Verification items for the finished model (mm, model axes). A direction names the side the tool comes from. Round coordinates to 2 decimals unless told otherwise and drop trailing zeros. Loops run counter-clockwise (first coordinate to the right, second up) from the corner with the lowest first, then second, coordinate; pieces in that order, holes last. Notation, with made-up numbers: (32, -36.5) -> (87, -36.5) arc R20 ccw to (87, -24.5) -> close; hole circle Ø11 at (-14, -1). An arc over 180 degrees is marked (long way). Write item = value, one per line. Start each with the question number.
```python
from build123d import *

# Parameters (mm, degrees)
SKETCH2_R           = 15
SKETCH2_R_2         = 11
BOSS_EXTRUDE1_DEPTH = 9
BOSS_EXTRUDE2_DEPTH = 9
SKETCH4_W           = 12.7
SKETCH4_H           = 16
BOSS_EXTRUDE3_DEPTH = 3.8
SKETCH5_R           = 1.275
CUT_EXTRUDE1_DEPTH  = 7
SKETCH6_R           = 11
SKETCH6_R_2         = 8
BOSS_EXTRUDE4_DEPTH = 1.5
BOSS_EXTRUDE5_DEPTH = 9
SKETCH8_W           = 12
SKETCH8_H           = 2
SKETCH8_W_2         = 2
SKETCH8_H_2         = 12
CUT_EXTRUDE2_DEPTH  = 13.8
CUT_EXTRUDE3_REACH  = 34
SKETCH9_R           = 0.95
CUT_EXTRUDE4_REACH  = 48.456
SKETCH10_R          = 0.95
FILLET1_R           = 4
FILLET3_R           = 2
SKETCH11_R          = 11
BOSS_EXTRUDE6_DEPTH = 1.5
SKETCH13_R          = 0.95
CUT_EXTRUDE5_DEPTH  = 9
FILLET2_R           = 1


with BuildPart() as part:
    # Sketch2 → Boss-Extrude1 (new body)
    with BuildSketch(Plane.XY):
        Circle(SKETCH2_R)
        Circle(SKETCH2_R_2, mode=Mode.SUBTRACT)
    extrude(amount=BOSS_EXTRUDE1_DEPTH)

    # Sketch3 → Boss-Extrude2 (add)
    with BuildSketch(Plane.XY):
        with BuildLine():
            Line((-6.35, -13.589610002), (-6.35, -33.589610002))
            Line((-6.35, -33.589610002), (6.35, -33.589610002))
            Line((6.35, -33.589610002), (6.35, -13.589610002))
            ThreePointArc((6.35, -13.589610002), (0, -15), (-6.35, -13.589610002))
        make_face()
    extrude(amount=BOSS_EXTRUDE2_DEPTH)

    # Sketch4 → Boss-Extrude3 (add)
    with BuildSketch(Plane.XY):
        with Locations((0, -25.589610002)):
            Rectangle(SKETCH4_W, SKETCH4_H)
    extrude(amount=-BOSS_EXTRUDE3_DEPTH)

    # Sketch5 → Cut-Extrude1 (cut)
    with BuildSketch(Plane.XZ.offset(33.589610002)):
        with Locations((0, 2.6)):
            Circle(SKETCH5_R)
    extrude(amount=-CUT_EXTRUDE1_DEPTH, mode=Mode.SUBTRACT)

    # Sketch6 → Boss-Extrude4 (add)
    with BuildSketch(Plane.XY.offset(9)):
        Circle(SKETCH6_R)
        Circle(SKETCH6_R_2, mode=Mode.SUBTRACT)
    extrude(amount=-BOSS_EXTRUDE4_DEPTH)

    # Sketch7 → Boss-Extrude5 (add)
    with BuildSketch(Plane.XY):
        Polygon((-2, 14.866068747), (2, 10.866068747), (32, 10.866068747), (32, 14.866068747), (2, 14.866068747), (2, 31), (-2, 31), align=None)
    extrude(amount=BOSS_EXTRUDE5_DEPTH)

    # Sketch8 → Cut-Extrude2 (cut, through all)
    with BuildSketch(Plane.XY.offset(9)):
        with Locations((26, 13.866068747)):
            Rectangle(SKETCH8_W, SKETCH8_H)
        with Locations((-1, 25)):
            Rectangle(SKETCH8_W_2, SKETCH8_H_2)
    extrude(amount=-CUT_EXTRUDE2_DEPTH, mode=Mode.SUBTRACT)

    # Sketch9 → Cut-Extrude3 (cut, up to next)
    with BuildSketch(Plane.ZY, mode=Mode.PRIVATE) as cut_extrude3_sk1:
        with Locations((4.5, 27.5)):
            Circle(SKETCH9_R)
    cut_extrude3_tool1 = extrude(cut_extrude3_sk1.sketch, amount=-CUT_EXTRUDE3_REACH, mode=Mode.PRIVATE) & part.part
    add(cut_extrude3_tool1.solids().sort_by_distance((0, 27.5, 4.5))[0], mode=Mode.SUBTRACT)
    # Sketch9 → Cut-Extrude3 (cut, up to next)
    with BuildSketch(Plane.ZY, mode=Mode.PRIVATE) as cut_extrude3_sk2:
        with Locations((4.5, 22.5)):
            Circle(SKETCH9_R)
    cut_extrude3_tool2 = extrude(cut_extrude3_sk2.sketch, amount=-CUT_EXTRUDE3_REACH, mode=Mode.PRIVATE) & part.part
    add(cut_extrude3_tool2.solids().sort_by_distance((0, 22.5, 4.5))[0], mode=Mode.SUBTRACT)

    # Sketch10 → Cut-Extrude4 (cut, up to next)
    with BuildSketch(Plane(origin=(0, 12.866068747, 0), x_dir=(1, 0, 0), z_dir=(0, 1, 0)), mode=Mode.PRIVATE) as cut_extrude4_sk1:
        with Locations((23.5, -4.5)):
            Circle(SKETCH10_R)
    cut_extrude4_tool1 = extrude(cut_extrude4_sk1.sketch, amount=-CUT_EXTRUDE4_REACH, mode=Mode.PRIVATE) & part.part
    add(cut_extrude4_tool1.solids().sort_by_distance((23.5, 12.866069, 4.5))[0], mode=Mode.SUBTRACT)
    # Sketch10 → Cut-Extrude4 (cut, up to next)
    with BuildSketch(Plane(origin=(0, 12.866068747, 0), x_dir=(1, 0, 0), z_dir=(0, 1, 0)), mode=Mode.PRIVATE) as cut_extrude4_sk2:
        with Locations((28.5, -4.5)):
            Circle(SKETCH10_R)
    cut_extrude4_tool2 = extrude(cut_extrude4_sk2.sketch, amount=-CUT_EXTRUDE4_REACH, mode=Mode.PRIVATE) & part.part
    add(cut_extrude4_tool2.solids().sort_by_distance((28.5, 12.866069, 4.5))[0], mode=Mode.SUBTRACT)

    # Fillet1
    fillet1_edges = [part.edges().sort_by_distance(p)[0] for p in [
        (2, 14.866068747, 4.5),
    ]]
    fillet(fillet1_edges, radius=FILLET1_R)

    # Fillet3
    fillet3_edges = [part.edges().sort_by_distance(p)[0] for p in [
        (-2, 14.866068747, 4.5),
    ]]
    fillet(fillet3_edges, radius=FILLET3_R)


with BuildPart() as body_2:
    # Sketch11 → Boss-Extrude6 (new body)
    with BuildSketch(Plane(origin=(0, 0, 0), x_dir=(-1, 0, 0), z_dir=(0, 0, -1))):
        with BuildLine():
            Line((-6, 14.866068747), (-10.340626189, 10.866068747))
            ThreePointArc((-10.340626189, 10.866068747), (-14.804198945, -2.415718027), (-6.35, -13.589610002))
            Line((-6.35, -13.589610002), (-6.35, -17.589610002))
            Line((-6.35, -17.589610002), (6.35, -17.589610002))
            Line((6.35, -17.589610002), (6.35, -13.589610002))
            ThreePointArc((6.35, -13.589610002), (14.92536147, 1.49451831), (3.529411765, 14.578863213))
            ThreePointArc((3.529411765, 14.578863213), (2.428189504, 15.286017757), (2, 16.522711642))
            Line((2, 16.522711642), (2, 19))
            Line((2, 19), (0, 19))
            Line((0, 19), (-2, 19))
            Line((-2, 19), (-2, 18.866068747))
            ThreePointArc((-2, 18.866068747), (-3.171572875, 16.037641623), (-6, 14.866068747))
        make_face()
        Circle(SKETCH11_R, mode=Mode.SUBTRACT)
    extrude(amount=BOSS_EXTRUDE6_DEPTH)


with BuildPart() as cut_extrude5_tool:
    # Sketch13 → Cut-Extrude5 (new body)
    with BuildSketch(Plane(origin=(0, 0, -1.5), x_dir=(-1, 0, 0), z_dir=(0, 0, -1))):
        with Locations((0, 15)):
            Circle(SKETCH13_R)
        with Locations((0, -15)):
            Circle(SKETCH13_R)
    extrude(amount=-CUT_EXTRUDE5_DEPTH)


with BuildPart() as part_1:
    add(part.part)

    # Cut-Extrude5: cut by cut_extrude5_tool
    add(cut_extrude5_tool.part, mode=Mode.SUBTRACT)


with BuildPart() as body_2_1:
    add(body_2.part)

    # Cut-Extrude5: cut by cut_extrude5_tool
    add(cut_extrude5_tool.part, mode=Mode.SUBTRACT)

    # Fillet2
    fillet2_edges = [body_2_1.edges().sort_by_distance(p)[0] for p in [
        (0, 19, -1.5),
    ]]
    fillet(fillet2_edges, radius=FILLET2_R)


solid = part_1.part
```
(1) Section check D-D on x = 23.5. Enter the section's corners in (y, z), then the cut area to 3 significant figures.
(2) Access from +Z, -Z, +X, -X, +Y, -Y to the whole of each face (thin tool, end or side, straight path). Record for faces 1 (the cylindrical face through (0.124, -14.058, 3.698)), 2 (the flat face through (0, -17.59, -2)), 3 (the flat face through (20, 14, 5)).
(3) Section check B-B on y = 0. Enter the section's corners in (x, z).
(4) Section check C-C on y = -15. Enter the section's corners in (x, z), then the cut area to 3 significant figures.
(5) Scan lines: line 1 (Z direction, x = 0, y = -32) (3 decimals); line 2 (Y direction, x = 1.55, z = 4.5); line 3 (Y direction, x = 1, z = 4.5). Record each from-to range of solid material in increasing order. Write a range as [from, to].
(6) Draft check along Y on faces 4 (the cylindrical face through (0.986, 26.573, 4.294)), 5 (the flat face through (0, 15, 7.5)), 6 (the flat face through (13, 14.866, 4)), 7 (the flat face through (2, 25, 4)). Enter one of: +Y half, -Y half, draft (parallel to the pull), parting line (faces both ways), or undercut.
(7) Section check A-A on x = 12. Enter the section's corners in (y, z).
(8) Depth check by flat-ended pin: pin 1 Ø4 at (x, z) = (22, 3) entering from -Y; pin 2 Ø6 at (x, y) = (-2, 12) entering from -Z; pin 3 Ø6 at (x, z) = (13, 0) entering from -Y. Enter the tip coordinate at first touch or a pass-through.
Computed values:
q1.outline = (10.87, 0) -> (12.87, 0) -> (12.87, 3.55) -> (10.87, 3.55) -> close; (10.87, 5.45) -> (12.87, 5.45) -> (12.87, 9) -> (10.87, 9) -> close
q1.area = 14.2 mm²
q2.face_1 = -Z
q2.face_2 = -Z, +X, -X, +Y
q2.face_3 = +Z, -Z, +X, +Y
q3.outline = (-15, 0) -> (-11, 0) -> (-11, 7.5) -> (-8, 7.5) -> (-8, 9) -> (-15, 9) -> close; (8, 7.5) -> (11, 7.5) -> (11, 0) -> (15, 0) -> (15, 9) -> (8, 9) -> close
q4.outline = (-6.35, 0) -> (-0.95, 0) -> (-0.95, 7.5) -> (0.95, 7.5) -> (0.95, 0) -> (6.35, 0) -> (6.35, 9) -> (-6.35, 9) -> close
q4.area = 100 mm²
q5.line_1 = [-3.8, 1.325], [3.875, 9]
q5.line_2 = [-33.59, -10.89], [10.89, 21.55], [23.45, 26.55], [28.45, 31]
q5.line_3 = [-33.59, -10.95], [10.95, 21.55], [23.45, 26.55], [28.45, 31]
q6.face_4 = undercut
q6.face_5 = undercut
q6.face_6 = +Y half
q6.face_7 = draft
q7.outline = (-9, 0) -> (9, 0) -> (9, 9) -> (-9, 9) -> close; (10.87, 0) -> (14.87, 0) -> (14.87, 9) -> (10.87, 9) -> close
q8.pin_1 = 10.87
q8.pin_2 = 0
q8.pin_3 = -11.18
